from build123d import *

# Parameters (mm, degrees)
F1_DEPTH  = 38.1
F2_W      = 53.239736706
F2_H      = 40.1604212821
F3_DEPTH  = 50.8
F4_R      = 17.5474664262
F5_DEPTH  = 38.1
F9_D      = 12.7
F10_R     = 6.6436508829
F11_DEPTH = 127


# Not quite as in the source:
# - a feature of the source that left no trace in its solid (it failed there, or was rolled back) is left out


with BuildPart() as f1:
    # F0 (on Front) → F1 (new body, symmetric)
    with BuildSketch(Plane.XZ):
        with BuildLine():
            ThreePointArc((-17.5968260456, 40.1604212821), (0, 22.5635952364), (17.5968260456, 40.1604212821))
            ThreePointArc((17.5968260456, 40.1604212821), (0, 57.7572473277), (-17.5968260456, 40.1604212821))
        make_face()
        with BuildLine():
            ThreePointArc((-17.5968260456, 0), (0, -17.5968260456), (17.5968260456, 0))
            ThreePointArc((17.5968260456, 0), (0, 17.5968260456), (-17.5968260456, 0))
        make_face()
        with BuildLine():
            ThreePointArc((-17.5968260456, 0), (0, 17.5968260456), (17.5968260456, 0))
            Line((17.5968260456, 0), (17.5968260456, 40.1604212821))
            ThreePointArc((17.5968260456, 40.1604212821), (0, 22.5635952364), (-17.5968260456, 40.1604212821))
            Line((-17.5968260456, 40.1604212821), (-17.5968260456, 0))
        make_face()
    extrude(amount=F1_DEPTH, both=True)

    # F2 (on face) → F3 (cut)
    with BuildSketch(Plane.YZ.offset(17.5968260456)):
        Polygon((0, 66.9256597757), (-26.619868353, 66.9256597757), (-26.619868353, 40.1604212821), (26.619868353, 40.1604212821), (26.619868353, 66.9256597757), align=None)
        with Locations((0, 20.080210641)):
            Rectangle(F2_W, F2_H)
        Polygon((26.619868353, 0), (-26.619868353, 0), (-26.619868353, -26.9206576049), (0, -26.9206576049), (26.619868353, -26.9206576049), align=None)
    extrude(amount=-F3_DEPTH, mode=Mode.SUBTRACT)

    # F4 (on Front) → F5 (join, symmetric)
    with BuildSketch(Plane.XZ):
        Circle(F4_R)
    extrude(amount=F5_DEPTH, both=True)

    # F9 (through all)
    with Locations(Plane.XZ.offset(38.1)):
        with Locations((0, 0)):
            Hole(F9_D / 2)

    # F10 (on face) → F11 (cut)
    with BuildSketch(Plane(origin=(0, 38.1, 0), x_dir=(-1, 0, 0), z_dir=(0, 1, 0))):
        with Locations((0, 42.4637757242)):
            Circle(F10_R)
    extrude(amount=-F11_DEPTH, mode=Mode.SUBTRACT)


solid = f1.part
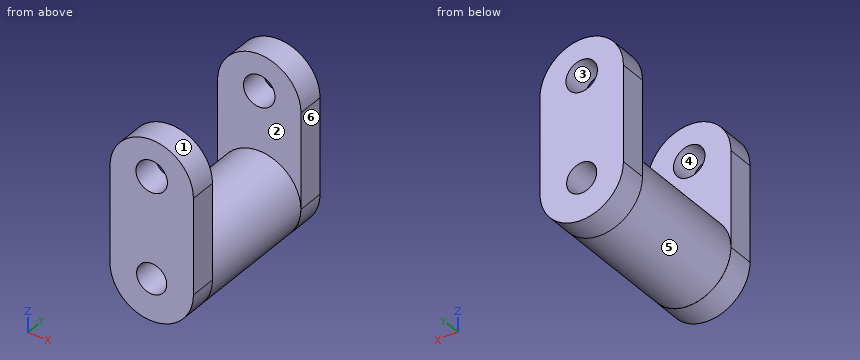
Design review of the part built by this model. Coordinates are the model's own, in mm. Face numbers are marked on the shaded views. A direction names the side the tool comes from. Coordinates: 2 decimals unless noted, no trailing zeros. Loops run counter-clockwise (first coordinate to the right, second up) from the corner with the lowest first, then second, coordinate; pieces in that order, holes last. Notation, with made-up numbers: (38.5, 49.25) -> (59.5, 49.25) arc R17 ccw to (59.5, 73.25) -> close; hole circle Ø8 at (1, -14). An arc over 180 degrees is marked (long way). Use a Markdown table: item, result. Add a question column.
Item 1: We need section A-A, the plane x = 0. Write out the cut boundary in (y, z), and give its area (3 significant figures).
Item 2: We need section B-B, the plane z = 3. Write out the cut boundary in (x, y).
Item 3: We need section C-C, the plane y = 15. Write out the cut boundary in (x, z), and give its area (3 significant figures).
Item 4: Machinability: for the marked faces 5 and 6, which of the approach directions +Z, -Z, +X, -X, +Y, -Y give a long, thin tool a straight path to every point of the face, cutting with its end or side? Answer none if there is none.
Item 5: Wall thickness on L1, parallel to Z at x = 0, y = 32.5; L2, parallel to Y at x = -6, z = 24; L3, parallel to Z at x = 0, y = 17: over which ranges is each line inside the solid? List them lowest first. Write a range as from..to.
Item 6: We need section D-D, the plane y = 30. Write out the cut boundary in (x, z), and give its area (3 significant figures).
Item 7: Clearance check with flat-ended pins moving along their axes: P1, Ø1, axis at x = 12.5, y = 13.5, coming from the -Z side; P2, Ø1, axis at y = 24.5, z = 2, coming from the +X side; P3, Ø10.5, axis at x = 0, z = 42.46, coming from the -Y side; P4, Ø8, axis at y = -24, z = 47, coming from the -X side. State where each tip first meets the part, or that it passes through.
Item 8: The part is to be moulded in two halves that separate along Z. For the marked faces 1, 2, 3 and 4, say which applies: +Z half, -Z half, draft (parallel to the pull), parting line (faces both ways), or undercut.
Numbers:
| question | item | result |
|---|---|---|
| 1 | outline | (-38.1, -17.6) -> (-26.62, -17.6) -> (-26.62, -17.55) -> (26.62, -17.55) -> (26.62, -17.6) -> (38.1, -17.6) -> (38.1, -6.35) -> (-38.1, -6.35) -> close; (-38.1, 6.35) -> (38.1, 6.35) -> (38.1, 35.82) -> (26.62, 35.82) -> (26.62, 17.55) -> (-26.62, 17.55) -> (-26.62, 35.82) -> (-38.1, 35.82) -> close; (-38.1, 49.11) -> (-26.62, 49.11) -> (-26.62, 57.76) -> (-38.1, 57.76) -> close; (26.62, 49.11) -> (38.1, 49.11) -> (38.1, 57.76) -> (26.62, 57.76) -> close |
| 1 | area | 2,330 mm^2 |
| 2 | outline | (-17.6, -38.1) -> (-5.6, -38.1) -> (-5.6, 38.1) -> (-17.6, 38.1) -> (-17.6, 26.62) -> (-17.29, 26.62) -> (-17.29, -26.62) -> (-17.6, -26.62) -> close; (5.6, -38.1) -> (17.6, -38.1) -> (17.6, -26.62) -> (17.29, -26.62) -> (17.29, 26.62) -> (17.6, 26.62) -> (17.6, 38.1) -> (5.6, 38.1) -> close |
| 3 | outline | circle Ø35.09 at (0, 0); hole circle Ø12.7 at (0, 0) |
| 3 | area | 841 mm^2 |
| 4 | face 5 | none |
| 4 | face 6 | +Z, -Z, +X, +Y, -Y |
| 5 | L1 | z = -17.6..-6.35, 6.35..35.82, 49.11..57.76 |
| 5 | L2 | y = -38.1..-26.62, 26.62..38.1 |
| 5 | L3 | z = -17.55..-6.35, 6.35..17.55 |
| 6 | outline | (-17.6, 0) arc R17.6 ccw to (17.6, 0) -> (17.6, 40.16) arc R17.6 ccw to (-17.6, 40.16) -> close; hole circle Ø13.29 at (0, 42.46); hole circle Ø12.7 at (0, 0) |
| 6 | area | 2,120 mm^2 |
| 7 | P1 | stops at z = -12.8 |
| 7 | P2 | stops at x = 17.48 |
| 7 | P3 | passes through |
| 7 | P4 | stops at x = -17.18 |
| 8 | face 1 | +Z half |
| 8 | face 2 | draft |
| 8 | face 3 | undercut |
| 8 | face 4 | undercut |
